Geometry check sheet. Reference: the model listing, model coordinates, mm. A direction names the side the tool comes from. Round coordinates to 2 decimals unless told otherwise and drop trailing zeros.
from build123d import *

# Parameters (mm, degrees)
SKETCH_1_W                   = 55
SKETCH_1_H                   = 145
EXTRUDE_1_DEPTH              = 12
HOLE_WIZARD_M3_1_D           = 3.5
HOLE_WIZARD_M3_1_CBORE_D     = 6
HOLE_WIZARD_M3_1_CBORE_DEPTH = 5
HOLE_WIZARD_1_D              = 4.5
HOLE_WIZARD_1_CBORE_D        = 8
HOLE_WIZARD_1_CBORE_DEPTH    = 5
HOLE_WIZARD_M5_1_D           = 4.2
HOLE_WIZARD_M5_1_DEPTH       = 14
HOLE_WIZARD_M5_1_TIP         = 1.2618073
HOLE_WIZARD_M3_1_2_D         = 2.5
HOLE_WIZARD_M3_1_2_DEPTH     = 8.5
HOLE_WIZARD_M3_1_2_TIP       = 0.751075774
CHAMFER_1_SIZE               = 1


with BuildPart() as part:
    # 草图1 → 凸台-拉伸1 (new body)
    with BuildSketch(Plane.XY):
        with Locations((-24.869961125, -27.624351889)):
            Rectangle(SKETCH_1_W, SKETCH_1_H)
    extrude(amount=EXTRUDE_1_DEPTH)

    # Hole Wizard M3 _1 (through all)
    with Locations(Plane.XY.offset(12)):
        with Locations((-32.369961125, 37.875648111), (-17.369961125, 37.875648111), (-17.369961125, 17.875648111), (-32.369961125, 17.875648111)):
            hole_wizard_m3_1 = CounterBoreHole(HOLE_WIZARD_M3_1_D / 2, HOLE_WIZARD_M3_1_CBORE_D / 2, HOLE_WIZARD_M3_1_CBORE_DEPTH)

    # 镜向1: Hole Wizard M3 _1 across plane
    add(hole_wizard_m3_1.mirror(Plane.ZX.offset(-27.624351889)), mode=Mode.SUBTRACT)

    # 打孔尺寸(%根据)内六角圆柱头螺钉的类型1 (through all)
    with Locations(Plane(origin=(27.369961125, 27.624351889, 12), x_dir=(1, 0, 0), z_dir=(0, 0, 1))):
        with Locations((-74.73992225, -40.748703777), (-54.73992225, -40.748703777), (-34.73992225, -40.748703777), (-34.73992225, -69.748703777), (-54.73992225, -69.748703777), (-74.73992225, -69.748703777)):
            CounterBoreHole(HOLE_WIZARD_1_D / 2, HOLE_WIZARD_1_CBORE_D / 2, HOLE_WIZARD_1_CBORE_DEPTH)

    # M5 螺纹孔1
    with Locations(Plane.XY.offset(12)):
        with Locations((-47.369961125, 24.875648111), (-2.369961125, 24.875648111), (-2.369961125, -27.624351889), (-47.369961125, -27.624351889), (-47.369961125, -80.124351889), (-2.369961125, -80.124351889)):
            Hole(HOLE_WIZARD_M5_1_D / 2, depth=HOLE_WIZARD_M5_1_DEPTH)
            with Locations((0, 0, -(HOLE_WIZARD_M5_1_DEPTH + HOLE_WIZARD_M5_1_TIP / 2))):  # 118° drill point
                Cone(0, HOLE_WIZARD_M5_1_D / 2, HOLE_WIZARD_M5_1_TIP, mode=Mode.SUBTRACT)

    # Hole Wizard M3 _1 2
    with Locations(Plane(origin=(0, 0, 0), x_dir=(-1, 0, 0), z_dir=(0, 0, -1))):
        with Locations((29.369961125, -61.124351889), (20.369961125, -61.124351889)):
            Hole(HOLE_WIZARD_M3_1_2_D / 2, depth=HOLE_WIZARD_M3_1_2_DEPTH)
            with Locations((0, 0, -(HOLE_WIZARD_M3_1_2_DEPTH + HOLE_WIZARD_M3_1_2_TIP / 2))):  # 118° drill point
                Cone(0, HOLE_WIZARD_M3_1_2_D / 2, HOLE_WIZARD_M3_1_2_TIP, mode=Mode.SUBTRACT)

    # 倒角1
    chamfer_1_edges = [part.edges().sort_by_distance(p)[0] for p in [
        (-52.369961125, 44.875648111, 6),
        (2.630038875, 44.875648111, 6),
        (2.630038875, -100.124351889, 6),
        (-52.369961125, -100.124351889, 6),
    ]]
    chamfer(chamfer_1_edges, length=CHAMFER_1_SIZE)


solid = part.part
1. Depth check by flat-ended pin: pin 1 Ø1.8 at (x, y) = (-32.5, 39) entering from +Z; pin 2 Ø2.5 at (x, y) = (-27.37, -13.12) entering from -Z. Enter the tip coordinate at first touch or a pass-through.
2. Scan lines: line 1 along X through (y, z) = (-42.5, 7.5); line 2 along Y through (x, z) = (-4.5, 9.75); line 3 along Y through (x, z) = (-1, 6.5). Record each from-to range of solid material in increasing order.
3. Release check for a two-part mould opening along X. For faces 1 (the face through (-25, -27, 12)), 2 (the face through (-34.04, 18.4, 3.45)), 3 (the face through (2.63, -29, 6)) record: +X half, -X half, draft (parallel to the pull), parting line (faces both ways), or undercut.
4. Section check A-A (x = -48). State how many separate pieces and enclosed holes the cut face has, plus the area to 3 significant figures.
5. Access from +Z, -Z, +X, -X, +Y, -Y to the whole of each face (thin tool, end or side, straight path). Record for faces 4 (the face through (-30.99, -90.46, 9.54)), 5 (the face through (-3.339, -29.487, 5.916)).
Results below:
1. pin 1: stops at z = 7
1. pin 2: passes through
2. line 1: x = -52.37 to -51.35, -43.39 to -31.35, -23.39 to -11.35, -3.39 to 2.63
2. line 2: y = -100.12 to -44.91, -39.34 to -15.91, -10.34 to 44.88
2. line 3: y = -100.12 to -81.72, -78.53 to -29.22, -26.03 to 23.28, 26.47 to 44.88
3. face 1: draft
3. face 2: undercut
3. face 3: +X half
4. separate pieces: 6
4. enclosed holes: 0
4. area: 1,460 mm2
5. face 4: +Z
5. face 5: +Z, -Z
